from build123d import *

# Parameters (mm, degrees)
SKETCH_2_R          = 4
CUT_EXTRUDE_1_DEPTH = 124.36


with BuildPart() as part:
    # 草图1 → 旋转1 (revolve)
    with BuildSketch(Plane.XY):
        Polygon((73.298050743, 37), (42.698050743, 37), (42.698050743, 35.9), (2.578050743, 35.9), (2.578050743, 37), (-40.061949257, 37), (-40.061949257, 59.300299501), (-50.061949257, 59.300299501), (-50.061949257, 31.28), (-9.061949257, 31.28), (-9.061949257, 29.28), (54.338050743, 29.28), (54.338050743, 31.28), (73.298050743, 31.28), align=None)
    revolve(axis=Axis((-67.043189493, 0, 0), (1, 0, 0)))

    # 草图2 → 切除-拉伸1 (cut, through all)
    with BuildSketch(Plane.ZY.offset(50.061949257)):
        with Locations((0, 43.5)):
            Circle(SKETCH_2_R)
        with Locations((43.5, 0)):
            Circle(SKETCH_2_R)
        with Locations((0, -43.5)):
            Circle(SKETCH_2_R)
        with Locations((-43.5, 0)):
            Circle(SKETCH_2_R)
    extrude(amount=-CUT_EXTRUDE_1_DEPTH, mode=Mode.SUBTRACT)


solid = part.part
Input: part model. Units: mm. Frame: model coordinates. A direction names the side the tool comes from. Give positions to 0.01 mm unless a question says otherwise; leave off trailing zeros. Order: outer loops, then holes, each group sorted by start corner. A loop starts at its lowest first (then second) coordinate and runs counter-clockwise, first axis right, second up.
Q1. Contact query for flat-ended pins moving along their axis: pin 1 Ø4 at (x, y) = (23.5, -31.5) entering from +Z; pin 2 Ø3 at (x, y) = (-8, -12.5) entering from -Z; pin 3 Ø7 at (y, z) = (0, -43.5) entering from -X; pin 4 Ø1 at (x, y) = (-14.5, -12) entering from -Z. Output: stop coordinate, or through.
Checked values:
pin 1: stops at z = 20.46
pin 2: stops at z = -35.33
pin 3: passes through
pin 4: stops at z = -35.17
Q2. Draft query along Y for faces 1 (the flat face through (-50.062, 26, -26)), 2 (the cylindrical face through (57.78, -8.02, -36.12)), 3 (the cylindrical face through (63.951, 29.836, 9.396)). Return one class per face: +Y half, -Y half, draft (parallel to the pull), parting line (faces both ways), or undercut.
Checked values:
face 1: draft
face 2: parting line
face 3: undercut
Q3. Section D-D on y = 0. State how many separate pieces and enclosed holes the cut face has, and give its area (3 significant figures).
Checked values:
separate pieces: 4
enclosed holes: 0
area: 1,860 mm2
Q4. Section B-B on z = 42. Output: boundary loops of the cut face in (x, y), and give its area (3 significant figures).
Checked values:
outline: (-50.06, -41.86) - (-40.06, -41.86) - (-40.06, -3.71) - (-50.06, -3.71) - close; (-50.06, 3.71) - (-40.06, 3.71) - (-40.06, 41.86) - (-50.06, 41.86) - close
area: 763 mm2
Q5. Ray query, probe 1 along Y at (x, z) = (47, 0.5); probe 2 along Z at (x, y) = (-18, 0); probe 3 along X at (y, z) = (-32.5, 19). Return the intervals inside material, ascending.
Checked values:
probe 1: y = -37 to -29.28, 29.28 to 37
probe 2: z = -37 to -31.28, 31.28 to 37
probe 3: x = -50.06 to -40.06
Q6. Section A-A on y = 26. Output: boundary loops of the cut face in (x, z) (3 decimals), and give its area (3 significant figures).
Checked values:
outline: (-50.062, -53.297) - (-40.062, -53.297) - (-40.062, -26.325) - (2.578, -26.325) - (2.578, -24.755) - (42.698, -24.755) - (42.698, -26.325) - (73.298, -26.325) - (73.298, -17.391) - (54.338, -17.391) - (54.338, -13.465) - (-9.062, -13.465) - (-9.062, -17.391) - (-50.062, -17.391) - close; (-50.062, 17.391) - (-9.062, 17.391) - (-9.062, 13.465) - (54.338, 13.465) - (54.338, 17.391) - (73.298, 17.391) - (73.298, 26.325) - (42.698, 26.325) - (42.698, 24.755) - (2.578, 24.755) - (2.578, 26.325) - (-40.062, 26.325) - (-40.062, 53.297) - (-50.062, 53.297) - close
area: 3,120 mm2
Q7. Set-up query: faces 4 (the cylindrical face through (-29.275, 29.836, 9.396)), 5 (the flat face through (42.698, -3, 36)), 6 (the flat face through (-40.062, 1, -39)). Return all of +Z, -Z, +X, -X, +Y, -Y with unobstructed straight access to the full face (end or side cutting, diameter ignored); none if empty.
Checked values:
face 4: -X
face 5: none
face 6: +X
Q8. Section C-C on x = 16.5. Output: boundary loops of the cut face in (y, z).
Checked values:
outline: circle Ø71.8 at (0, 0); hole circle Ø58.56 at (0, 0)
